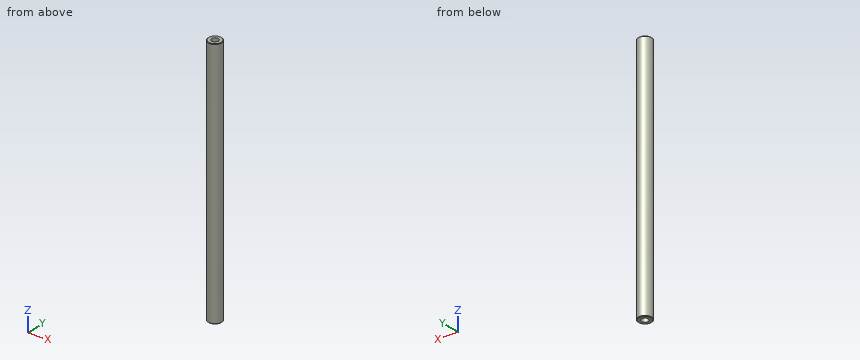
Autodesk Inventor part; units mm, degrees
ref_plane "YZ Plane" through (0, 0, 0) normal (1, 0, 0) x (0, 1, 0)
ref_plane "XZ Plane" through (0, 0, 0) normal (0, 1, 0) x (-1, 0, 0)
ref_plane "XY Plane" through (0, 0, 0) normal (0, 0, 1) x (1, 0, 0)
sketch "Sketch1" plane through (0, 0, 0) normal (0, 0, 1) x (1, 0, 0)
  circle A0 centre (0, 0) radius 6
  dimension "d0" = 12
extrude "Extrusion1" add sketch "Sketch1" along normal mid plane 220
sketch "Sketch2" plane through (0, 0, -110) normal (0, 0, -1) x (-1, 0, 0)
  point P0 (0, 0)
  point P1 (0, 0)
hole "Hole1" at (0, 0, -110) direction (0, 0, 1) diameter 6 depth 20 tip angle 118
thread "Thread1"
mirror "Mirror1" about plane through (0, 0, 0) normal (0, 0, 1) of "Hole1"
chamfer "Chamfer2" distance 0.5 angle 45 2 edges at (-6, 0, -110) (-6, 0, 110)
properties part number "Rod-12x220-M6" material "Stainless Steel"
Read the model definition and answer for the solid it produces. Units are mm, in the model's axes. Coordinates: 2 decimals unless noted, no trailing zeros. Loops run counter-clockwise (first coordinate to the right, second up) from the corner with the lowest first, then second, coordinate; pieces in that order, holes last. Notation, with made-up numbers: (-26.75, 27) -> (-0.75, 27) arc R15 cw to (-0.75, 35) -> close; hole circle Ø10 at (12.25, 5.25). An arc over 180 degrees is marked (long way). Answer in a Markdown table with one row per item.
Item 1: A cutting plane is placed at A-A on z = -19. Determine the outline of the cut face in (x, y), plus the area to 3 significant figures.
Returned:
| item | result |
|---|---|
| outline | circle Ø12 at (0, 0) |
| area | 113 mm^2 |
Item 2: Each of these flat-tipped pins is pushed along its axis until it touches: P1, Ø3.5, axis at x = 0, y = 0, coming from the -Z side; P2, Ø2, axis at y = -1.5, z = 44.5, coming from the +X side; P3, Ø1.5, axis at y = -2, z = 88, coming from the -X side. Where does it stop, or does it pass through?
Returned:
| item | result |
|---|---|
| P1 | stops at z = -89.25 |
| P2 | stops at x = 5.98 |
| P3 | stops at x = -5.87 |
Item 3: Straight lines are drawn through the part: line 1 along Y through (x, z) = (0, 99.25); line 2 along Y through (x, z) = (5, 99); line 3 along Y through (x, z) = (-3.5, -96). For each, find the intervals that lie inside material, in ascending order. Write a range as [from, to].
Returned:
| item | result |
|---|---|
| line 1 | y = [-6, -3], [3, 6] |
| line 2 | y = [-3.32, 3.32] |
| line 3 | y = [-4.87, 4.87] |
